Build history of the part. All positions in model axes, mm. Face numbers are marked on the shaded views. A direction names the side the tool comes from. Coordinates: 2 decimals unless noted, no trailing zeros. Order: outer loops, then holes, each group sorted by start corner. A loop starts at its lowest first (then second) coordinate and runs counter-clockwise, first axis right, second up. Notation, with made-up numbers: (-26.75, 30.5) - (12.25, 30.5) arc R21 ccw to (12.25, 69.5) - close; hole circle Ø9 at (32.25, 57.25). An arc over 180 degrees is marked (long way). One line per item, written item: value.
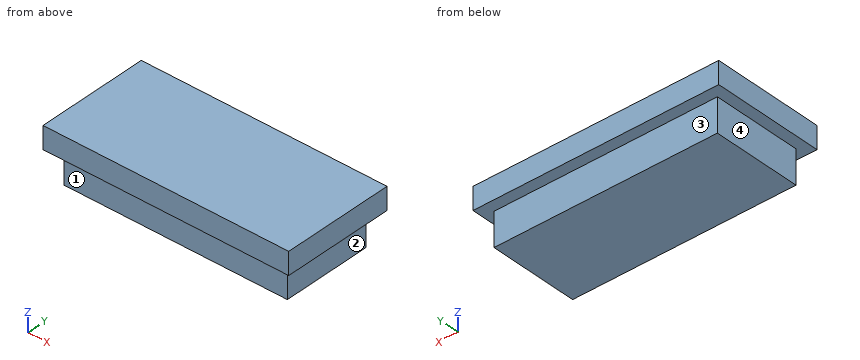
from build123d import *

# Parameters (mm, degrees)
SKETCH1_W           = 12.7
SKETCH1_H           = 5.08
BOSS_EXTRUDE1_DEPTH = 1.27
SKETCH2_W           = 13.97
SKETCH2_H           = 6.35
BOSS_EXTRUDE2_DEPTH = 0.635


with BuildPart() as part:
    # Sketch1 → Boss-Extrude1 (new, symmetric)
    with BuildSketch(Plane.XY):
        Rectangle(SKETCH1_W, SKETCH1_H)
    extrude(amount=BOSS_EXTRUDE1_DEPTH, both=True)

    # Sketch2 → Boss-Extrude2 (add, symmetric)
    with BuildSketch(Plane.XY.offset(1.27)):
        Rectangle(SKETCH2_W, SKETCH2_H)
    extrude(amount=BOSS_EXTRUDE2_DEPTH, both=True)


solid = part.part
1. Band-saw the part on B-B, the plane x = 6. Give the cut face in (y, z) (3 decimals), and give its area (3 significant figures).
Values found:
outline: (-3.175, 0.635) - (-2.54, 0.635) - (-2.54, -1.27) - (2.54, -1.27) - (2.54, 0.635) - (3.175, 0.635) - (3.175, 1.905) - (-3.175, 1.905) - close
area: 17.7 mm2
2. Probe line 1 along X through (y, z) = (-0.5, -0.5); line 2 along Y through (x, z) = (3.5, 0.4); line 3 along Z through (x, y) = (-2.5, 2.75) (3 decimals). List the from-to ranges inside material, lowest first.
Values found:
line 1: x = -6.35 to 6.35
line 2: y = -2.54 to 2.54
line 3: z = 0.635 to 1.905
3. 3-axis set-ups, long thin cutter, end or side, ignore diameter. For the marked faces 1, 2, 3 and 4: which of +Z, -Z, +X, -X, +Y, -Y reach the whole face in a straight line?
Values found:
face 1: -Z, +X, -X, -Y
face 2: -Z, +X, +Y, -Y
face 3: -Z, +X, -X, +Y
face 4: -Z, -X, +Y, -Y
4. Band-saw the part on C-C, the plane z = 0.45. Give the cut face in (x, y).
Values found:
outline: (-6.35, -2.54) - (6.35, -2.54) - (6.35, 2.54) - (-6.35, 2.54) - close
5. Band-saw the part on A-A, the plane y = 1.25. Give the cut face in (x, z) (3 decimals).
Values found:
outline: (-6.985, 0.635) - (-6.35, 0.635) - (-6.35, -1.27) - (6.35, -1.27) - (6.35, 0.635) - (6.985, 0.635) - (6.985, 1.905) - (-6.985, 1.905) - close
6. Flat gauge pins, fed straight in: P1, Ø1.5, axis at x = 0.5, z = -0.5, coming from the +Y side; P2, Ø0.6, axis at y = -1, z = -0.5, coming from the +X side; P3, Ø1.5, axis at x = 1.5, z = -0.5, coming from the -Y side. Where does each tip first touch, or does it go through?
Values found:
P1: stops at y = 2.54
P2: stops at x = 6.35
P3: stops at y = -2.54
